The listing builds one solid part. Answer for the finished solid, in the listing's coordinates (mm). Round coordinates to 2 decimals unless told otherwise and drop trailing zeros. Order: outer loops, then holes, each group sorted by start corner. A loop starts at its lowest first (then second) coordinate and runs counter-clockwise, first axis right, second up. Notation, with made-up numbers: (-9, 32) - (14, 32) arc R31 cw to (14, 64) - close; hole circle Ø11 at (28.25, 49). An arc over 180 degrees is marked (long way). One line per item, written item: value. Start each with the question number.
1. Section C-C, the plane z = -145 is taken. Give the vertices of the cut face in (x, y) (3 decimals), then the cut area to 3 significant figures.
2. Section B-B, the plane x = 695.5 is taken. Give the vertices of the cut face in (y, z) (3 decimals).
3. Straight lines are drawn through the part: line 1 (X direction, y = 1.85, z = -527.05) (3 decimals); line 2 (Z direction, x = 162.5, y = 2.3) (3 decimals); line 3 (Z direction, x = 58, y = 1.25). For each, find the intervals that lie inside material, in ascending order.
4. A flat-ended cylindrical pin translates along its axis: P1, Ø4, axis at x = 170.83, z = -6.35, coming from the -Y side. Find the tip coordinate at first contact, or state that the pin passes through.
5. Section A-A, the plane y = 0.7 is taken. Count the separate pieces of the cut face and the enclosed holes in it, then the cut area to 3 significant figures.
from build123d import *

# Parameters (mm, degrees)
BOSS_EXTRUDE1_DEPTH         = 3.175
FILLET1_R                   = 3.175
F_1_4_0_25_DIAMETER_HOLE1_D = 6.35
SKETCH5_R                   = 3.175
CUT_EXTRUDE1_DEPTH          = 1016.052018679


with BuildPart() as part:
    # Sketch1 → Boss-Extrude1 (new body)
    with BuildSketch(Plane(origin=(0, 0, 0), x_dir=(1, 0, 0), z_dir=(0, 1, 0))):
        Polygon((0, 0), (352.425, 0), (863.6, 468.405587878), (863.6, 533.4), (0, 533.4), align=None)
    extrude(amount=BOSS_EXTRUDE1_DEPTH)

    # Fillet1
    fillet1_edges = [part.edges().sort_by_distance(p)[0] for p in [
        (0, 1.5875, -533.4),
        (863.6, 1.5875, -533.4),
        (863.6, 1.5875, -468.405587878),
        (352.425, 1.5875, 0),
        (0, 1.5875, 0),
    ]]
    fillet(fillet1_edges, radius=FILLET1_R)

    # 1/4 (0.25) Diameter Hole1 (through all)
    with Locations(Plane(origin=(0, 3.175, 0), x_dir=(1, 0, 0), z_dir=(0, 1, 0))):
        with Locations((43.832655013, 6.35), (170.832655013, 6.35), (297.832655013, 6.35), (414.05335701, 65.084754558), (620.048644915, 253.844658566), (826.043932819, 442.604562573), (50.8, 527.05), (431.8, 527.05), (812.8, 527.05)):
            Hole(F_1_4_0_25_DIAMETER_HOLE1_D / 2)

    # Sketch5 → Cut-Extrude1 (cut, through all)
    with BuildSketch(Plane(origin=(0, 3.175, 0), x_dir=(1, 0, 0), z_dir=(0, 1, 0))):
        with Locations(Location((297.832655013, 6.35, 0), (0, 0, 270))):
            Circle(SKETCH5_R)
        with Locations(Location((170.832655013, 6.35, 0), (0, 0, 270))):
            Circle(SKETCH5_R)
        with Locations(Location((43.832655013, 6.35, 0), (0, 0, 270))):
            Circle(SKETCH5_R)
        with BuildLine():
            Line((31.132655013, 34.925), (56.532655013, 34.925))
            ThreePointArc((56.532655013, 34.925), (66.057655013, 25.4), (56.532655013, 15.875))
            Line((56.532655013, 15.875), (31.132655013, 15.875))
            ThreePointArc((31.132655013, 15.875), (21.607655013, 25.4), (31.132655013, 34.925))
        make_face()
        with BuildLine():
            Line((158.132655013, 34.925), (183.532655013, 34.925))
            ThreePointArc((183.532655013, 34.925), (193.057655013, 25.4), (183.532655013, 15.875))
            Line((183.532655013, 15.875), (158.132655013, 15.875))
            ThreePointArc((158.132655013, 15.875), (148.607655013, 25.4), (158.132655013, 34.925))
        make_face()
        with BuildLine():
            Line((285.132655013, 34.925), (310.532655013, 34.925))
            ThreePointArc((310.532655013, 34.925), (320.057655013, 25.4), (310.532655013, 15.875))
            Line((310.532655013, 15.875), (285.132655013, 15.875))
            ThreePointArc((285.132655013, 15.875), (275.607655013, 25.4), (285.132655013, 34.925))
        make_face()
    extrude(amount=-CUT_EXTRUDE1_DEPTH, mode=Mode.SUBTRACT)


solid = part.part
Answer list:
1. outline: (0, 0) - (510.665, 0) - (510.665, 3.175) - (0, 3.175) - close
1. area: 1,620 mm²
2. outline: (0, -533.4) - (3.175, -533.4) - (3.175, -314.37) - (0, -314.37) - close
3. line 1: x = 0 to 47.625, 53.975 to 428.625, 434.975 to 809.625, 815.975 to 863.6
3. line 2: z = -533.4 to -34.925, -15.875 to 0
3. line 3: z = -533.4 to -34.81, -15.99 to 0
4. P1: passes through
5. separate pieces: 1
5. enclosed holes: 12
5. area: 338,000 mm²
